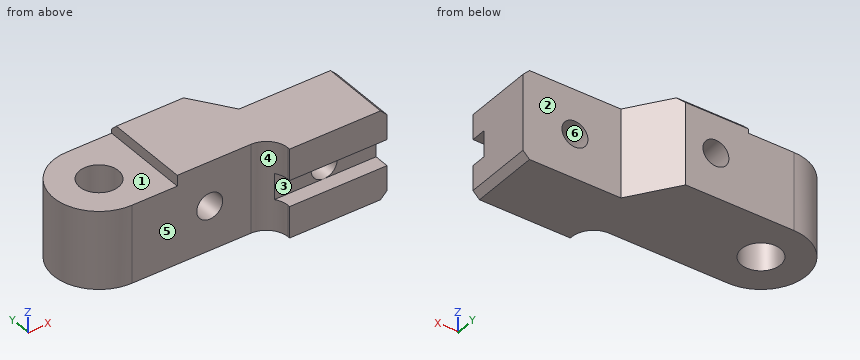
from build123d import *

# Parameters (mm, degrees)
SKETCH1_R           = 21
SKETCH1_R_2         = 9
BOSS_EXTRUDE1_DEPTH = 20.5
SKETCH2_R           = 6
SKETCH2_W           = 42
SKETCH2_H           = 5
CUT_EXTRUDE1_DEPTH  = 55
SKETCH3_W           = 12
SKETCH3_H           = 7
CUT_EXTRUDE2_DEPTH  = 55
CHAMFER1_SIZE       = 3


with BuildPart() as part:
    # Sketch1 → Boss-Extrude1 (new, symmetric)
    # profile 1 of 2: a face of its own
    with BuildSketch(Plane.XY):
        with BuildLine():
            Line((50, 21), (0, 21))
            ThreePointArc((0, 21), (14.849242405, 14.849242405), (21, 0))
            ThreePointArc((21, 0), (14.849242405, -14.849242405), (0, -21))
            Line((0, -21), (55, -21))
            ThreePointArc((55, -21), (62.071067812, -23.928932188), (65, -31))
            Line((65, -31), (65, -32))
            Line((65, -32), (110, -32))
            Line((110, -32), (110, 0))
            Line((110, 0), (64.704358302, 0))
            Line((64.704358302, 0), (50, 21))
        make_face()
    # profile 2 of 2: a face of its own
    with BuildSketch(Plane.XY):
        Circle(SKETCH1_R)
        Circle(SKETCH1_R_2, mode=Mode.SUBTRACT)
    extrude(amount=BOSS_EXTRUDE1_DEPTH, both=True)

    # Sketch2 → Cut-Extrude1 (cut)
    with BuildSketch(Plane(origin=(0, 21, 0), x_dir=(1, 0, 0), z_dir=(0, 1, 0))):
        with Locations(Location((36, 0, 0), (0, 0, 180))):
            Circle(SKETCH2_R)
        with Locations(Location((86, 0, 0), (0, 0, 270))):
            Circle(SKETCH2_R)
        with Locations((0, -18)):
            Rectangle(SKETCH2_W, SKETCH2_H)
    extrude(amount=-CUT_EXTRUDE1_DEPTH, mode=Mode.SUBTRACT)

    # Sketch3 → Cut-Extrude2 (cut)
    with BuildSketch(Plane(origin=(110, 0, 0), x_dir=(0, 0, -1), z_dir=(1, 0, 0))):
        with Locations((0, -28.5)):
            Rectangle(SKETCH3_W, SKETCH3_H)
    extrude(amount=-CUT_EXTRUDE2_DEPTH, mode=Mode.SUBTRACT)

    # Chamfer1
    chamfer1_edges = [part.edges().sort_by_distance(p)[0] for p in [
        (110, -16, -20.5),
        (110, -16, 20.5),
        (35.5, 21, 20.5),
    ]]
    chamfer(chamfer1_edges, length=CHAMFER1_SIZE)


solid = part.part
Geometry: final body of the model. Coordinates: model frame, mm. Face numbers are marked on the shaded views. A direction names the side the tool comes from. Give positions to 0.01 mm unless a question says otherwise; leave off trailing zeros. Write each loop counter-clockwise with the first axis right and the second up, starting at its lowest first coordinate (ties: lowest second). Pieces come first, ordered by that corner, then holes. Notation, with made-up numbers: (9.5, 42) - (47.5, 42) arc R24 ccw to (47.5, 64) - close; hole circle Ø7 at (70.25, -16). An arc over 180 degrees is marked (long way). Return JSON: item names as keys, results as strings. Group by question number.
1) Section C-C on y = -6. Return the cut outline in (x, z), plus the area to 3 significant figures.
2) Mould query, pull axis X, two halves, no side actions, for the marked faces 4, 5 and 6. Classes: released by +X, released by -X, zero draft, split by the parting line, or undercut.
3) Line query: line 1 (Z direction, x = 36, y = -5); line 2 (X direction, y = -12.5, z = 0.5); line 3 (Y direction, x = 31, z = -5.5). Output: solid intervals per line, ascending.
4) Set-up query: the marked faces 1, 2 and 3. Return all of +Z, -Z, +X, -X, +Y, -Y with unobstructed straight access to the full face (end or side cutting, diameter ignored); none if empty.
5) Section D-D on y = 3. Return the cut outline in (x, z), plus the area to 3 significant figures.
6) Section A-A on x = 36. Return the cut outline in (y, z), plus the area to 3 significant figures.
7) Section B-B on z = -4. Return the cut outline in (x, y).
8) First-contact query: P1, Ø19, axis at x = 86, z = 0, coming from the +Y side; P2, Ø0.8, axis at y = -31.5, z = -15, coming from the -X side; P3, Ø3, axis at y = 4.5, z = -6, coming from the -X side. Flat tips, straight axial feed; report the tip coordinate or a pass-through.
Filled in:
{
 "1": {"outline": "(-20.12, -20.5) - (-6.71, -20.5) - (-6.71, 15.5) - (-20.12, 15.5) - close; (6.71, -20.5) - (107, -20.5) - (110, -17.5) - (110, 17.5) - (107, 20.5) - (21, 20.5) - (21, 15.5) - (6.71, 15.5) - close; hole circle Ø12 at (36, 0); hole circle Ø12 at (86, 0)", "area": "4,410 mm^2"},
 "2": {"face 4": "released by -X", "face 5": "zero draft", "face 6": "undercut"},
 "3": {"line 1": "z = -20.5 to -6, 6 to 20.5", "line 2": "x = -16.87 to 30.02, 41.98 to 80.02, 91.98 to 110", "line 3": "y = -21 to 21"},
 "4": {"face 1": "+Z, -X, +Y, -Y", "face 2": "+Z, -Z, +X, +Y", "face 3": "+X, -X, -Y"},
 "5": {"outline": "(-20.78, -20.5) - (-8.49, -20.5) - (-8.49, 15.5) - (-20.78, 15.5) - close; (8.49, -20.5) - (62.6, -20.5) - (62.6, 20.5) - (21, 20.5) - (21, 15.5) - (8.49, 15.5) - close; hole circle Ø12 at (36, 0)", "area": "2,490 mm^2"},
 "6": {"outline": "(-21, -20.5) - (21, -20.5) - (21, -6) - (-21, -6) - close; (-21, 6) - (21, 6) - (21, 17.5) - (18, 20.5) - (-21, 20.5) - close", "area": "1,210 mm^2"},
 "7": {"outline": "(0, -21) - (31.53, -21) - (31.53, 21) - (0, 21) arc R21 ccw to start; (40.47, -21) - (55, -21) arc R10 cw to (63, -25) - (81.53, -25) - (81.53, 0) - (64.7, 0) - (50, 21) - (40.47, 21) - close; (90.47, -25) - (110, -25) - (110, 0) - (90.47, 0) - close; hole circle Ø18 at (0, 0)"},
 "8": {"P1": "stops at y = 0", "P2": "stops at x = 65", "P3": "stops at x = -20.78"}
}
